Check sheet for the drawn part. Datum: minimum x, y, z corner. Units: mm. A direction names the side the tool comes from. Give positions to 0.01 mm unless a question says otherwise; leave off trailing zeros. Order: outer loops, then holes, each group sorted by start corner. A loop starts at its lowest first (then second) coordinate and runs counter-clockwise, first axis right, second up.
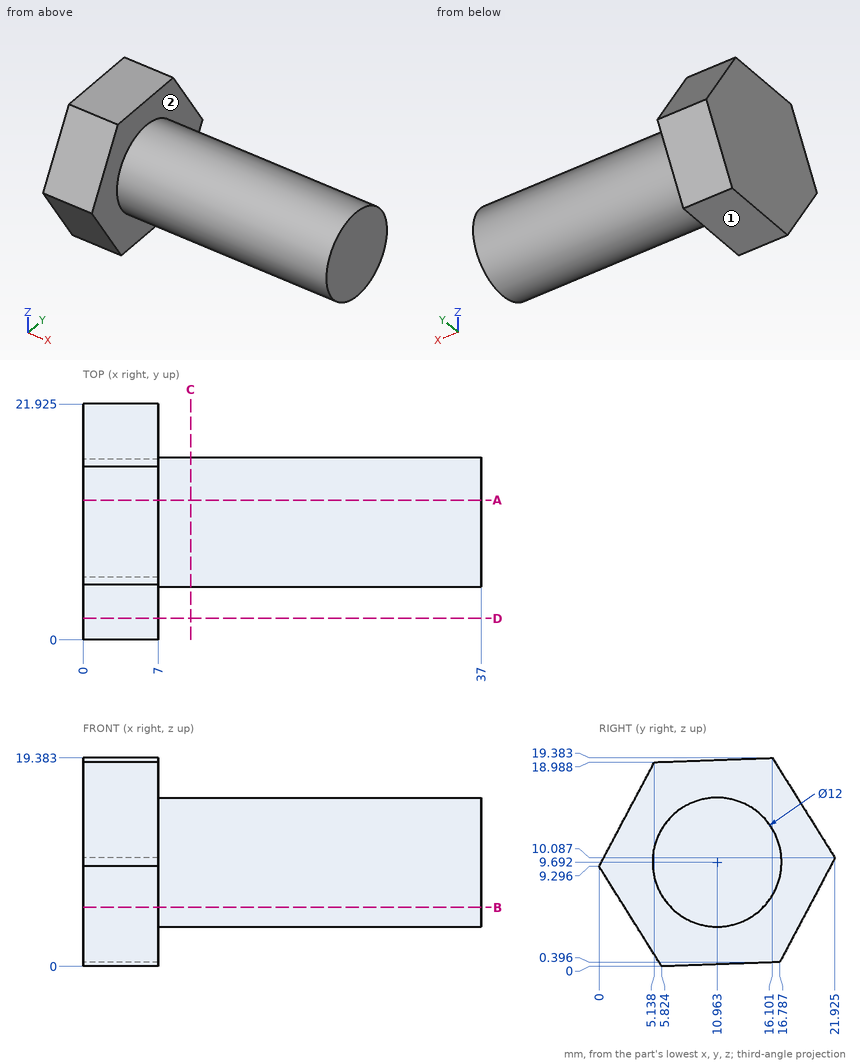
(1) Section check C-C, the plane x = 10. Enter the section's corners in (y, z), then the cut area to 3 significant figures.
Solved:
outline: circle Ø12 at (10.96, 9.69)
area: 113 mm2
(2) Go/stop test with flat-tipped pins: pin 1 (5 mm diameter, centred on y = 4, z = 13.5, fed in from +X); pin 2 (10 mm diameter, centred on x = 21.5, y = 13.5, fed in from -Z); pin 3 (4 mm diameter, centred on x = 19.5, z = 10, fed in from -Y); pin 4 (4 mm diameter, centred on x = 27.5, z = 5, fed in from +Y) (1 decimal). Record where each tip stops, or that it passes through.
Solved:
pin 1: stops at x = 37
pin 2: stops at z = 3.69
pin 3: stops at y = 4.96
pin 4: stops at y = 16.3
(3) Section check D-D, the plane y = 2. Enter the section's corners in (x, z).
Solved:
outline: (0, 6.1) - (7, 6.1) - (7, 13.07) - (0, 13.07) - close
(4) Section check A-A, the plane y = 13. Enter the section's corners in (x, z) (1 decimal).
Solved:
outline: (0, 0.3) - (7, 0.3) - (7, 4) - (37, 4) - (37, 15.3) - (7, 15.3) - (7, 19.3) - (0, 19.3) - close
(5) Scan lines: line 1 (X direction, y = 15.75, z = 15); line 2 (Y direction, x = 26.5, z = 10) (1 decimal); line 3 (Z direction, x = 25.5, y = 8.75) (1 decimal). Record each from-to range of solid material in increasing order.
Solved:
line 1: x = 0 to 7
line 2: y = 5 to 17
line 3: z = 4.1 to 15.3
(6) Section check B-B, the plane z = 5.5. Enter the section's corners in (x, y) (1 decimal), then the cut area to 3 significant figures.
Solved:
outline: (0, 2.4) - (7, 2.4) - (7, 6.7) - (37, 6.7) - (37, 15.3) - (7, 15.3) - (7, 19.5) - (0, 19.5) - close
area: 377 mm2
(7) Set-up check for the marked faces 1 and 2: record each of +Z, -Z, +X, -X, +Y, -Y from which the full face is reachable in a straight line by a thin tool's end or side.
Solved:
face 1: -Z, +X, -X, +Y
face 2: +X
